Here's how the part is built. I have some questions about the finished solid (model axes, mm). A direction names the side the tool comes from. Round coordinates to 2 decimals unless told otherwise and drop trailing zeros. Order: outer loops, then holes, each group sorted by start corner. A loop starts at its lowest first (then second) coordinate and runs counter-clockwise, first axis right, second up. Notation, with made-up numbers: (71, 57.5) -> (122, 57.5) arc R17 ccw to (122, 72.5) -> close; hole circle Ø4 at (-0.75, 22.5). An arc over 180 degrees is marked (long way). Answer in a Markdown table with one row per item.
```python
from build123d import *

# Parameters (mm, degrees)
SKETCH_1_R               = 20
EXTRUDE_1_DEPTH          = 5
EXTRUDE_2_DEPTH          = 8
FILLET_1_R               = 0.5
PATTERN_START            = 5
PATTERN_CIRCULAR_1_DEPTH = 8
SKETCH_3_R               = 2.5000000000000004
CUT_EXTRUDE_1_DEPTH      = 5
EXTRUDE_START            = 4.5
SKETCH_3_3_R             = 2.5000000000000004
SKETCH_3_3_R_2           = 2.2999999999999994
EXTRUDE_3_DEPTH          = 4.5
CHAMFER_1_SIZE           = 0.5
SKETCH_4_R               = 2.75
CUT_EXTRUDE_2_DEPTH      = 34.26033673912518
CHAMFER_2_SIZE           = 2


# Read off the part's stored shape, not the designer's step: 阵列(圆周)1
with BuildPart() as part:
    # 草图1 → 凸台-拉伸1 (new body)
    with BuildSketch(Plane(origin=(0, 0, 0), x_dir=(1, 0, 0), z_dir=(0, 1, 0))):
        with Locations(Location((0, 0, 0), (0, 0, 270))):
            Circle(SKETCH_1_R)
    extrude(amount=EXTRUDE_1_DEPTH)

    # 草图2 → 凸台-拉伸2 (add)
    with BuildSketch(Plane(origin=(0, 5, 0), x_dir=(1, 0, 0), z_dir=(0, 1, 0))):
        with BuildLine():
            Line((14.57106781186547, -7.500000000000001), (11.035533905932741, -3.9644660940672627))
            Line((11.035533905932741, -3.9644660940672627), (3.9644660940672627, -11.03553390593274))
            Line((3.9644660940672627, -11.03553390593274), (7.500000000000001, -14.571067811865477))
            Line((7.500000000000001, -14.571067811865477), (7.500000000000001, -18.540496217739157))
            ThreePointArc((7.500000000000001, -18.540496217739157), (14.142135623730951, -14.14213562373095), (18.540496217739157, -7.500000000000001))
            Line((18.540496217739157, -7.500000000000001), (14.57106781186547, -7.500000000000001))
        make_face()
    extrude(amount=EXTRUDE_2_DEPTH)

    # 圆角1
    fillet_1_edges = [part.edges().sort_by_distance(p)[0] for p in [
        (7.500000000000001, 9, 14.571067811865477),
        (7.500000000000001, 9, 18.540496217739157),
        (18.540496217739154, 9, 7.500000000000002),
        (14.57106781186547, 9, 7.500000000000001),
        (11.035533905932741, 9, 3.9644660940672627),
        (3.9644660940672627, 9, 11.03553390593274),
    ]]
    fillet(fillet_1_edges, radius=FILLET_1_R)

    # 阵列(圆周)1 outline → 阵列(圆周)1 (add)
    with BuildSketch(Plane(origin=(0, 0, 0), x_dir=(1, 0, 0), z_dir=(0, 1, 0)).offset(PATTERN_START)):
        with BuildLine():
            ThreePointArc((17.783419244, 7.5), (18.203278805, 7.728489505), (18.239404353, 8.205128205))
            ThreePointArc((18.239404353, 8.205128205), (14.142135624, 14.142135624), (8.205128205, 18.239404353))
            ThreePointArc((8.205128205, 18.239404353), (7.728489505, 18.203278805), (7.5, 17.783419244))
            Line((7.5, 17.783419244), (7.5, 14.778174593))
            ThreePointArc((7.5, 14.778174593), (7.461939766, 14.586832877), (7.353553391, 14.424621202))
            Line((7.353553391, 14.424621202), (4.318019485, 11.389087297))
            ThreePointArc((4.318019485, 11.389087297), (4.171572875, 11.035533906), (4.318019485, 10.681980515))
            Line((4.318019485, 10.681980515), (10.681980515, 4.318019485))
            ThreePointArc((10.681980515, 4.318019485), (11.035533906, 4.171572875), (11.389087297, 4.318019485))
            Line((11.389087297, 4.318019485), (14.424621202, 7.353553391))
            ThreePointArc((14.424621202, 7.353553391), (14.586832877, 7.461939766), (14.778174593, 7.5))
            Line((14.778174593, 7.5), (17.783419244, 7.5))
        make_face()
        with BuildLine():
            ThreePointArc((-18.239404353, -8.205128205), (-14.142135624, -14.142135624), (-8.205128205, -18.239404353))
            ThreePointArc((-8.205128205, -18.239404353), (-7.728489505, -18.203278805), (-7.5, -17.783419244))
            Line((-7.5, -17.783419244), (-7.5, -14.778174593))
            ThreePointArc((-7.5, -14.778174593), (-7.461939766, -14.586832877), (-7.353553391, -14.424621202))
            Line((-7.353553391, -14.424621202), (-4.318019485, -11.389087297))
            ThreePointArc((-4.318019485, -11.389087297), (-4.171572875, -11.035533906), (-4.318019485, -10.681980515))
            Line((-4.318019485, -10.681980515), (-10.681980515, -4.318019485))
            ThreePointArc((-10.681980515, -4.318019485), (-11.035533906, -4.171572875), (-11.389087297, -4.318019485))
            Line((-11.389087297, -4.318019485), (-14.424621202, -7.353553391))
            ThreePointArc((-14.424621202, -7.353553391), (-14.586832877, -7.461939766), (-14.778174593, -7.5))
            Line((-14.778174593, -7.5), (-17.783419244, -7.5))
            ThreePointArc((-17.783419244, -7.5), (-18.203278805, -7.728489505), (-18.239404353, -8.205128205))
        make_face()
        with BuildLine():
            ThreePointArc((-7.5, 17.783419244), (-7.728489505, 18.203278805), (-8.205128205, 18.239404353))
            ThreePointArc((-8.205128205, 18.239404353), (-14.142135624, 14.142135624), (-18.239404353, 8.205128205))
            ThreePointArc((-18.239404353, 8.205128205), (-18.203278805, 7.728489505), (-17.783419244, 7.5))
            Line((-17.783419244, 7.5), (-14.778174593, 7.5))
            ThreePointArc((-14.778174593, 7.5), (-14.586832877, 7.461939766), (-14.424621202, 7.353553391))
            Line((-14.424621202, 7.353553391), (-11.389087297, 4.318019485))
            ThreePointArc((-11.389087297, 4.318019485), (-11.035533906, 4.171572875), (-10.681980515, 4.318019485))
            Line((-10.681980515, 4.318019485), (-4.318019485, 10.681980515))
            ThreePointArc((-4.318019485, 10.681980515), (-4.171572875, 11.035533906), (-4.318019485, 11.389087297))
            Line((-4.318019485, 11.389087297), (-7.353553391, 14.424621202))
            ThreePointArc((-7.353553391, 14.424621202), (-7.461939766, 14.586832877), (-7.5, 14.778174593))
            Line((-7.5, 14.778174593), (-7.5, 17.783419244))
        make_face()
    extrude(amount=PATTERN_CIRCULAR_1_DEPTH)

    # 草图3 → 切除-拉伸1 (cut)
    with BuildSketch(Plane(origin=(0, 13.000000000000002, 0), x_dir=(1, 0, 0), z_dir=(0, 1, 0))):
        with Locations(Location((-10.681980515339466, 10.681980515339463, 0), (0, 0, 270))):
            Circle(SKETCH_3_R)
        with Locations(Location((10.681980515339466, -10.681980515339463, 0), (0, 0, 270))):
            Circle(SKETCH_3_R)
    extrude(amount=-CUT_EXTRUDE_1_DEPTH, mode=Mode.SUBTRACT)

    # 草图3<3> → 凸台-拉伸3 (add)
    with BuildSketch(Plane(origin=(0, 13.000000000000002, 0), x_dir=(1, 0, 0), z_dir=(0, 1, 0)).offset(EXTRUDE_START)):
        with Locations(Location((10.681980515339466, -10.681980515339463, 0), (0, 0, 270))):
            Circle(SKETCH_3_3_R)
        with Locations(Location((-10.681980515339466, 10.681980515339463, 0), (0, 0, 270))):
            Circle(SKETCH_3_3_R)
        with Locations(Location((10.681980515339466, 10.681980515339463, 0), (0, 0, 270))):
            Circle(SKETCH_3_3_R_2)
        with Locations(Location((-10.681980515339465, -10.681980515339465, 0), (0, 0, 270))):
            Circle(SKETCH_3_3_R_2)
    extrude(amount=-EXTRUDE_3_DEPTH)


with BuildPart() as extrude_3_kept_piece:
    # of the separate pieces the step leaves, the one the design keeps (extrude_3_pieces_kept)
    add(part.part.solids().sort_by_distance((8.205128205, 5, 18.239404353))[0])

    # 倒角1
    chamfer_1_edges = [extrude_3_kept_piece.edges().sort_by_distance(p)[0] for p in [
        (-10.681980515339466, 8.000000000000002, -13.181980515339463),
        (-10.681980515339466, 13.000000000000002, -13.181980515339463),
        (10.681980515339466, 8.000000000000002, 8.181980515339463),
        (10.681980515339466, 13.000000000000002, 8.181980515339463),
        (10.681980515339466, 13.000000000000002, -12.981980515339462),
        (10.681980515339466, 17.5, -12.981980515339462),
        (-10.681980515339465, 13.000000000000002, 8.381980515339466),
        (-10.681980515339465, 17.5, 8.381980515339466),
    ]]
    chamfer(chamfer_1_edges, length=CHAMFER_1_SIZE)

    # 草图4 → 切除-拉伸2 (cut, through all)
    with BuildSketch(Plane.XZ):
        with Locations(Location((0, 0, 0), (0, 0, 270))):
            Circle(SKETCH_4_R)
    extrude(amount=-CUT_EXTRUDE_2_DEPTH, mode=Mode.SUBTRACT)

    # 倒角2
    chamfer_2_edges = [extrude_3_kept_piece.edges().sort_by_distance(p)[0] for p in [
        (6.12e-15, 0, -20),
    ]]
    chamfer(chamfer_2_edges, length=CHAMFER_2_SIZE)


solid = extrude_3_kept_piece.part
```
1. Suppose I cut it at D-D on y = 1.5. Write out the boundary of the cut face in (x, z), then the cut area to 3 significant figures.
Numbers:
| item | result |
|---|---|
| outline | circle Ø39 at (0, 0); hole circle Ø5.5 at (0, 0) |
| area | 1,170 mm2 |
2. We'd pull the mould along Z, two halves only. Please class faces 1 (the face through (-9.931, 10.528, -8.297)), 2 (the face through (-12.3, 13, -13.4)), 3 (the face through (-16, 9, 7.5)), 4 (the face through (5.86, 8.94, -12.93)): released by +Z, released by -Z, zero draft, split by the parting line, or undercut.
Numbers:
| item | result |
|---|---|
| face 1 | undercut |
| face 2 | zero draft |
| face 3 | undercut |
| face 4 | released by -Z |
3. Suppose I cut it at B-B on z = 0. Write out the boundary of the cut face in (x, y), then the cut area to 4 significant figures.
Numbers:
| item | result |
|---|---|
| outline | (-20, 2) -> (-18, 0) -> (-2.75, 0) -> (-2.75, 5) -> (-20, 5) -> close; (2.75, 0) -> (18, 0) -> (20, 2) -> (20, 5) -> (2.75, 5) -> close |
| area | 168.5 mm2 |
4. Suppose I cut it at A-A on x = 0. Write out the boundary of the cut face in (y, z).
Numbers:
| item | result |
|---|---|
| outline | (0, -18) -> (2, -20) -> (5, -20) -> (5, -2.75) -> (0, -2.75) -> close; (0, 2.75) -> (5, 2.75) -> (5, 20) -> (2, 20) -> (0, 18) -> close |
5. For faces 5 (the face through (-5.86, 8.94, 12.93)), 6 (the face through (0, 5, -5)), 7 (the face through (7.5, 9, -16)), which set-ups out of +Z, -Z, +X, -X, +Y, -Y let a thin tool reach every point of the face, with its end or its side?
Numbers:
| item | result |
|---|---|
| face 5 | +Z, +Y |
| face 6 | +Y |
| face 7 | -Z, +Y |
6. For pin 1 Ø2 at (y, z) = (5, -4.5) entering from +X; pin 2 Ø4.5 at (x, z) = (10.68, 10.68) entering from +Y; pin 3 Ø4 at (x, z) = (-12.5, -11.5) entering from +Y; pin 4 Ø2 at (y, z) = (15.5, -6) entering from +X, each with a flat end and sliding along its axis, tell me the tip position at first contact or that it passes through.
Numbers:
| item | result |
|---|---|
| pin 1 | stops at x = 19.69 |
| pin 2 | stops at y = 8.25 |
| pin 3 | stops at y = 13 |
| pin 4 | passes through |
7. Please list where these lines run through material, in increasing order: line 1 along Y through (x, z) = (-3, 16); line 2 along Z through (x, y) = (18, 11.5); line 3 along Z through (x, y) = (-6, 9.25).
Numbers:
| item | result |
|---|---|
| line 1 | y = 0 to 5 |
| line 2 | z = -8.72 to -7.55, 7.55 to 8.72 |
| line 3 | z = -13.07 to -9, 9 to 13.07 |
8. Suppose I cut it at C-C on y = 16. Write out the boundary of the cut face in (x, z), then the cut area to 3 significant figures.
Numbers:
| item | result |
|---|---|
| outline | circle Ø4.6 at (-10.68, 10.68); circle Ø4.6 at (10.68, -10.68) |
| area | 33.2 mm2 |
